For this review, take the finished solid that the model builds, in its own axes (mm). Give positions to 0.01 mm unless a question says otherwise; leave off trailing zeros. Order: outer loops, then holes, each group sorted by start corner. A loop starts at its lowest first (then second) coordinate and runs counter-clockwise, first axis right, second up. Notation, with made-up numbers: (52, 36) - (84, 36) arc R29 ccw to (84, 67) - close; hole circle Ø6 at (0.5, 34). An arc over 180 degrees is marked (long way). Put each result on its own line as item: value. Start each with the question number.
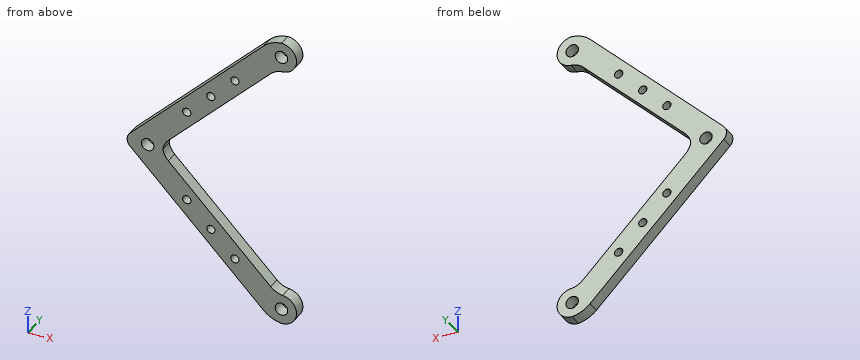
```python
from build123d import *

# Parameters (mm, degrees)
BOSS_EXTRUDE2_DEPTH = 6.35
SKETCH6_R           = 7.874
BOSS_EXTRUDE3_DEPTH = 6.35
CIRPATTERN1_COUNT   = 3
CIRPATTERN1_ANGLE   = 180
SKETCH7_R           = 2.15265
CUT_EXTRUDE1_DEPTH  = 118.095768176
FILLET1_R           = 15.24
FILLET2_R           = 10.16
FILLET3_R           = 5.08


with BuildPart() as part:
    # Sketch1 → Boss-Extrude2 (new body)
    with BuildSketch(Plane(origin=(0, 0, 0), x_dir=(1, 0, 0), z_dir=(0, 1, 0))):
        Polygon((-82.677748493, 0), (0, -82.677), (0, -64.716569057), (-64.71715495, 0), align=None)
    boss_extrude2 = extrude(amount=BOSS_EXTRUDE2_DEPTH)

    # Mirror1: Boss-Extrude2 across plane
    add(boss_extrude2.mirror(Plane.XY))

    # Sketch6 → Boss-Extrude3 (add)
    with BuildSketch(Plane(origin=(0, 6.35, 0), x_dir=(1, 0, 0), z_dir=(0, 1, 0))):
        with Locations((0, -69.85)):
            Circle(SKETCH6_R)
    boss_extrude3 = extrude(amount=-BOSS_EXTRUDE3_DEPTH)

    # Sketch5 → F (0.257) Diameter Hole1 (revolve, cut)
    with BuildSketch(Plane(origin=(0, 6.35, 69.85), x_dir=(0, 0, 1), z_dir=(1, 0, 0))):
        Polygon((0, 0), (0, 52.761148974), (3.2639, 50.8), (3.2639, 0), align=None)
    f_0_257_diameter_hole1 = revolve(axis=Axis((0, 12.7, 69.85), (0, -1, 0)), mode=Mode.SUBTRACT)

    # CirPattern1: Boss-Extrude3, F (0.257) Diameter Hole1 ×3 about axis
    cirpattern1_axis = Axis((0, 0, 0), (0, -1, 0))
    add([boss_extrude3.rotate(cirpattern1_axis, i * CIRPATTERN1_ANGLE / (CIRPATTERN1_COUNT - 1)) for i in range(1, CIRPATTERN1_COUNT)])
    add([f_0_257_diameter_hole1.rotate(cirpattern1_axis, i * CIRPATTERN1_ANGLE / (CIRPATTERN1_COUNT - 1)) for i in range(1, CIRPATTERN1_COUNT)], mode=Mode.SUBTRACT)

    # Sketch7 → Cut-Extrude1 (cut, through all)
    with BuildSketch(Plane(origin=(0, 6.35, 0), x_dir=(1, 0, 0), z_dir=(0, 1, 0))):
        with Locations(Location((-36.848766511, -36.848351615, 0), (0, 0, 270))):
            Circle(SKETCH7_R)
        with Locations(Location((-49.42112508, -24.275993045, 0), (0, 0, 270))):
            Circle(SKETCH7_R)
        with Locations(Location((-24.276407941, -49.420710184, 0), (0, 0, 270))):
            Circle(SKETCH7_R)
    cut_extrude1 = extrude(amount=-CUT_EXTRUDE1_DEPTH, mode=Mode.SUBTRACT)

    # Mirror2: Cut-Extrude1 across plane
    add(cut_extrude1.mirror(Plane.XY), mode=Mode.SUBTRACT)

    # Fillet1
    # the kernel refuses this fillet: 15.24 mm, written as the material it takes off along each edge
    with BuildSketch(Plane(origin=(0, -33.056477591, 82.677), x_dir=(-0.7071099819596415, 0, -0.707103580398965), z_dir=(0, 1, 0))) as fillet1_piece_1:
        with BuildLine():
            CenterArc((13.222591036, -15.24), FILLET1_R, 90, 39.629113094)
            Line((3.502284034, -3.502315741), (0, 0))
            Line((0, 0), (13.222591036, 0))
        make_face()
    extrude(amount=72.462955182, mode=Mode.SUBTRACT)
    with BuildSketch(Plane(origin=(0, -33.056477591, -82.677), x_dir=(-0.7071099819596415, 0, 0.707103580398965), z_dir=(0, 1, 0))) as fillet1_piece_2:
        with BuildLine():
            CenterArc((13.222591036, 15.24), FILLET1_R, 230.370886906, 39.629113094)
            Line((3.502284034, 3.502315741), (0, 0))
            Line((0, 0), (13.222591036, 0))
        make_face()
    extrude(amount=72.462955182, mode=Mode.SUBTRACT)

    # Fillet2
    # the kernel refuses this fillet: 10.16 mm, written as the material it adds along each edge
    with BuildSketch(Plane(origin=(-62.342579148, 0, 2.374554305), x_dir=(0.11040173938387075, 0, -0.9938870438540871), z_dir=(0, 1, 0))) as fillet2_piece_1:
        with BuildLine():
            CenterArc((5.03816312, -9.966042895), FILLET2_R, 101.213390693, 40.125343256)
            Line((-2.895302495, -3.618939355), (0, 0))
            ThreePointArc((0, 0), (1.531206438, -0.150316757), (3.062412877, 0))
        make_face()
    extrude(amount=6.35)
    with BuildSketch(Plane(origin=(-62.342579148, 0, -2.374554305), x_dir=(0.7071099819596407, 0, -0.7071035803989658), z_dir=(0, 1, 0))) as fillet2_piece_2:
        with BuildLine():
            CenterArc((4.634597997, -10.16), FILLET2_R, 90, 40.125343256)
            ThreePointArc((-1.913135001, -2.391294021), (-0.839192223, -1.289552131), (0, 0))
            Line((0, 0), (4.634597997, 0))
        make_face()
    extrude(amount=6.35)
    with BuildSketch(Plane(origin=(-2.374141848, 0, -62.342448702), x_dir=(0.9938916997559154, 0, 0.11035981676451387), z_dir=(0, 1, 0))) as fillet2_piece_3:
        with BuildLine():
            CenterArc((5.037838868, -9.966068103), FILLET2_R, 101.212659653, 40.12313883)
            Line((-2.895301552, -3.618558112), (0, 0))
            ThreePointArc((0, 0), (1.531107891, -0.150297221), (3.062215783, 0))
        make_face()
    extrude(amount=6.35)
    with BuildSketch(Plane(origin=(-2.374141848, 0, 62.342448702), x_dir=(-0.7071099819596428, 0, -0.7071035803989636), z_dir=(0, 1, 0))) as fillet2_piece_4:
        with BuildLine():
            CenterArc((4.634299719, -10.16), FILLET2_R, 90, 40.12313883)
            ThreePointArc((-1.913134377, -2.391042106), (-0.839211976, -1.289419981), (0, 0))
            Line((0, 0), (4.634299719, 0))
        make_face()
    extrude(amount=6.35)

    # Fillet3
    fillet3_edges = [part.edges().sort_by_distance(p)[0] for p in [
        (-82.677748493, 3.175, 0),
    ]]
    fillet(fillet3_edges, radius=FILLET3_R)


solid = part.part
```
1. Add section B-B, the plane z = -69.85. Give the boundary of the cut face in (x, y), then the cut area to 3 significant figures.
2. Add section C-C, the plane y = 2.5. Count the separate pieces of the cut face and the enclosed holes in it, then the cut area to 3 significant figures.
3. Add section D-D, the plane x = -63.5. Give the boundary of the cut face in (y, z), then the cut area to 3 significant figures.
4. Add section A-A, the plane x = -16.5. Give the boundary of the cut face in (y, z), then the cut area to 3 significant figures.
5. Wall thickness on line 1 (Z direction, x = -25, y = 1.75); line 2 (X direction, y = 6, z = 2); line 3 (Z direction, x = -71.5, y = 1): over which ranges is each line inside the solid? List them lowest first. Write a range as from..to.
6. Clearance check with flat-ended pins moving along their axes: pin 1 (3 mm diameter, centred on x = -44, y = 5, fed in from -Z); pin 2 (1.5 mm diameter, centred on y = 3.5, z = 42.5, fed in from +X). State where each tip first meets the part, or that it passes through.
Found:
1. outline: (-12.83, 0) - (-3.26, 0) - (-3.26, 6.35) - (-12.83, 6.35) - close; (3.26, 0) - (7.87, 0) - (7.87, 6.35) - (3.26, 6.35) - close
1. area: 90.0 mm^2
2. separate pieces: 1
2. enclosed holes: 9
2. area: 2,640 mm^2
3. outline: (0, -19.18) - (6.35, -19.18) - (6.35, 19.18) - (0, 19.18) - close
3. area: 244 mm^2
4. outline: (0, -66.18) - (6.35, -66.18) - (6.35, -48.22) - (0, -48.22) - close; (0, 48.22) - (6.35, 48.22) - (6.35, 66.18) - (0, 66.18) - close
4. area: 228 mm^2
5. line 1: z = -57.68..-51.45, -47.39..-39.72, 39.72..47.39, 51.45..57.68
5. line 2: x = -80.16..-72.43, -67.27..-61.41
5. line 3: z = -11.18..-2.82, 2.82..11.18
6. pin 1: stops at z = -40.18
6. pin 2: stops at x = -21.47
